Part model, mm, in its own coordinate system. Face numbers are marked on the shaded views. Give positions to 0.01 mm unless a question says otherwise; leave off trailing zeros. Order: outer loops, then holes, each group sorted by start corner. A loop starts at its lowest first (then second) coordinate and runs counter-clockwise, first axis right, second up. Notation, with made-up numbers: (-4.75, -5.75) - (12.25, -5.75) arc R22 ccw to (12.25, 1.25) - close; hole circle Ø8 at (2.5, -3). An arc over 180 degrees is marked (long way). Use a Markdown table: item, result. Add a question column.
from build123d import *

# Parameters (mm, degrees)
SKETCH1_R           = 2.25
BOSS_EXTRUDE1_DEPTH = 3.5
SKETCH2_W           = 8
SKETCH2_H           = 4
BOSS_EXTRUDE2_DEPTH = 30
CUT_EXTRUDE1_DEPTH  = 41.8
BOSS_EXTRUDE3_DEPTH = 8
FILLET3_R           = 0.5
FILLET4_R           = 1


with BuildPart() as part:
    # Sketch1 → Boss-Extrude1 (new body)
    with BuildSketch(Plane(origin=(0, 0, 0), x_dir=(1, 0, 0), z_dir=(0, 1, 0))):
        Polygon((0, 0), (81.7, 0), (81.7, 47.5), (85.842135624, 57.5), (81.7, 57.5), (0, 57.5), (-4.142135624, 57.5), (0, 47.5), align=None)
        with Locations((5, 5)):
            Circle(SKETCH1_R, mode=Mode.SUBTRACT)
        with Locations((76.7, 5)):
            Circle(SKETCH1_R, mode=Mode.SUBTRACT)
        with Locations((3.34089319, 52.5)):
            Circle(SKETCH1_R, mode=Mode.SUBTRACT)
        with Locations((78.35910681, 52.5)):
            Circle(SKETCH1_R, mode=Mode.SUBTRACT)
    extrude(amount=BOSS_EXTRUDE1_DEPTH)

    # Sketch2 → Boss-Extrude2 (add)
    with BuildSketch(Plane(origin=(0, 3.5, 0), x_dir=(1, 0, 0), z_dir=(0, 1, 0))):
        with Locations((4, 18.7)):
            Rectangle(SKETCH2_W, SKETCH2_H)
        with Locations((77.7, 18.7)):
            Rectangle(SKETCH2_W, SKETCH2_H)
    extrude(amount=BOSS_EXTRUDE2_DEPTH)

    # Sketch3 → Cut-Extrude1 (cut, through all)
    with BuildSketch(Plane.XY.offset(-16.7)):
        with BuildLine():
            Line((0.834660634, 28.15), (0, 28.15))
            Line((0, 28.15), (0, 26.15))
            Line((0, 26.15), (0.834660634, 26.15))
            ThreePointArc((0.834660634, 26.15), (6.25, 27.15), (0.834660634, 28.15))
        make_face()
        with BuildLine():
            Line((0, 10.85), (0.834660634, 10.85))
            ThreePointArc((0.834660634, 10.85), (6.25, 9.85), (0.834660634, 8.85))
            Line((0.834660634, 8.85), (0, 8.85))
            Line((0, 8.85), (0, 10.85))
        make_face()
        with BuildLine():
            Line((81.7, 8.85), (81.7, 10.85))
            Line((81.7, 10.85), (80.865339366, 10.85))
            ThreePointArc((80.865339366, 10.85), (75.45, 9.85), (80.865339366, 8.85))
            Line((80.865339366, 8.85), (81.7, 8.85))
        make_face()
        with BuildLine():
            Line((81.7, 26.15), (80.865339366, 26.15))
            ThreePointArc((80.865339366, 26.15), (75.45, 27.15), (80.865339366, 28.15))
            Line((80.865339366, 28.15), (81.7, 28.15))
            Line((81.7, 28.15), (81.7, 26.15))
        make_face()
    extrude(amount=-CUT_EXTRUDE1_DEPTH, mode=Mode.SUBTRACT)

    # Sketch4 → Boss-Extrude3 (add)
    with BuildSketch(Plane(origin=(0, 0, 0), x_dir=(0, 0, -1), z_dir=(1, 0, 0))):
        Polygon((20.7, 23.5), (40.7, 3.5), (35.7, 3.5), (20.7, 18.5), align=None)
    boss_extrude3 = extrude(amount=BOSS_EXTRUDE3_DEPTH)

    # Mirror1: Boss-Extrude3 across plane
    add(boss_extrude3.mirror(Plane(origin=(40.85, 0, 0), x_dir=(0, 0, 1), z_dir=(1, 0, 0))))

    # Fillet3
    fillet3_edges = [part.edges().sort_by_distance(p)[0] for p in [
        (80.865339366, 26.15, -18.7),
        (80.865339366, 28.15, -18.7),
        (0.834660634, 10.85, -18.7),
        (0.834660634, 8.85, -18.7),
        (0, 33.5, -18.7),
        (81.7, 33.5, -18.7),
        (0.834660634, 28.15, -18.7),
        (0.834660634, 26.15, -18.7),
        (80.865339366, 8.85, -18.7),
        (80.865339366, 10.85, -18.7),
    ]]
    fillet(fillet3_edges, radius=FILLET3_R)

    # Fillet4
    fillet4_edges = [part.edges().sort_by_distance(p)[0] for p in [
        (0, 1.75, -47.5),
        (-4.142135624, 1.75, -57.5),
        (85.842135624, 1.75, -57.5),
        (81.7, 1.75, -47.5),
        (81.7, 1.75, 0),
        (0, 1.75, 0),
    ]]
    fillet(fillet4_edges, radius=FILLET4_R)


solid = part.part
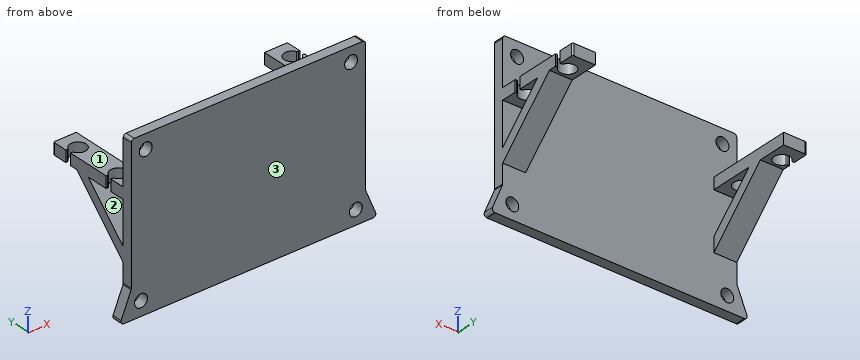
1. Mould opens along Y. For the marked faces 1, 2 and 3 say: released by +Y, released by -Y, zero draft, split by the parting line, or undercut.
2. Cut at C-C (x = 4.5). Write the cut outline in (y, z), plus the area to 3 significant figures.
3. Drill centre lines: probe 1 along Y at (x, z) = (3.45, -19.3); probe 2 along X at (y, z) = (1, -5); probe 3 along X at (y, z) = (1, -52). Where is each one in solid material? Low to high. Write a range as [from, to].
4. Cut at A-A (y = 9.85). Write the cut outline in (x, z).
5. Cut at D-D (z = -5). Write the cut outline in (x, y).
6. Pin check, flat tips, straight feed: P1, Ø6.5, axis at x = 78.5, y = 28, coming from the -Z side; P2, Ø3, axis at y = 31, z = -18.5, coming from the -X side; P3, Ø8, axis at x = 45, z = -51, coming from the +Y side. Stop position of each tip, or through.
7. Cut at B-B (z = -24.5). Write the cut outline in (x, y).
Responses:
| question | item | result |
|---|---|---|
| 1 | face 1 | zero draft |
| 1 | face 2 | undercut |
| 1 | face 3 | released by -Y |
| 2 | outline | (0, -57.5) - (3.5, -57.5) - (3.5, -54.43) - (0, -54.43) - close; (0, -50.57) - (3.5, -50.57) - (3.5, -40.7) - (23.5, -20.7) - (24.55, -20.7) - (24.55, -16.7) - (12.45, -16.7) - (12.45, -20.7) - (18.5, -20.7) - (3.5, -35.7) - (3.5, -20.7) - (7.25, -20.7) - (7.25, -16.7) - (3.5, -16.7) - (3.5, -7.19) - (0, -7.19) - close; (0, -2.81) - (3.5, -2.81) - (3.5, 0) - (0, 0) - close; (29.75, -20.7) - (33.5, -20.7) - (33.5, -16.7) - (29.75, -16.7) - close |
| 2 | area | 338 mm² |
| 3 | probe 1 | y = [0, 7.05], [12.65, 24.35], [29.95, 33.5] |
| 3 | probe 2 | x = [0, 2.75], [7.25, 74.45], [78.95, 81.7] |
| 3 | probe 3 | x = [-1.86, 1.15], [5.53, 76.17], [80.55, 83.56] |
| 4 | outline | (0, -34.35) - (8, -34.35) - (8, -29.35) - (0, -29.35) - close; (6.25, -20.7) - (8, -20.7) - (8, -16.7) - (6.25, -16.7) - close; (73.7, -34.35) - (81.7, -34.35) - (81.7, -29.35) - (73.7, -29.35) - close; (73.7, -20.7) - (75.45, -20.7) - (75.45, -16.7) - (73.7, -16.7) - close |
| 5 | outline | (0, 0) - (2.75, 0) - (2.75, 3.5) - (0, 3.5) - close; (7.25, 0) - (74.45, 0) - (74.45, 3.5) - (7.25, 3.5) - close; (78.95, 0) - (81.7, 0) - (81.7, 3.5) - (78.95, 3.5) - close |
| 6 | P1 | stops at z = -20.7 |
| 6 | P2 | stops at x = 0 |
| 6 | P3 | stops at y = 3.5 |
| 7 | outline | (0, 0) - (81.7, 0) - (81.7, 3.5) - (0, 3.5) - close; (0, 14.7) - (8, 14.7) - (8, 19.7) - (0, 19.7) - close; (73.7, 14.7) - (81.7, 14.7) - (81.7, 19.7) - (73.7, 19.7) - close |
